```python
from build123d import *
from build123d.topology import SkipClean

# Parameters (mm, degrees)
SKETCH_1_R           = 7.5
SKETCH_1_R_2         = 4.5
EXTRUDE_1_DEPTH      = 125
EXTRUDE_2_REACH      = 151.958
EXTRUDE_2_END_RADIUS = 7.5
SKETCH_2_R           = 7.5
SKETCH_2_R_2         = 4.5
EXTRUDE_3_REACH      = 169.5
EXTRUDE_3_END_RADIUS = 7.5
SKETCH_3_R           = 7.5
SKETCH_3_R_2         = 4.5
SKETCH_4_R           = 7.5
EXTRUDE_4_DEPTH      = 5
EXTRUDE_START        = 5
SKETCH_5_R           = 7.5
EXTRUDE_5_DEPTH      = 5


with BuildPart() as part:
    # 草图1 → 凸台-拉伸1 (new, symmetric)
    with BuildSketch(Plane.XY):
        Circle(SKETCH_1_R)
        Circle(SKETCH_1_R_2, mode=Mode.SUBTRACT)
    extrude(amount=EXTRUDE_1_DEPTH, both=True)

    # 凸台-拉伸2: up to this cylinder (the profile starts outside it)
    extrude_2_end = Plane(origin=(0, 0, -7.287868), z_dir=(0, 0, -1)) * Cylinder(EXTRUDE_2_END_RADIUS, 319.916, mode=Mode.PRIVATE)
    # 草图2 → 凸台-拉伸2 (add, up to the surface)
    with BuildSketch(Plane(origin=(0, 75, 0), x_dir=(1, 0, 0), z_dir=(0, 1, 0)), mode=Mode.PRIVATE) as extrude_2_sk1:
        with Locations(Location((0, 0, 0), (0, 0, 270))):
            Circle(SKETCH_2_R)
        with Locations(Location((0, 0, 0), (0, 0, 270))):
            Circle(SKETCH_2_R_2, mode=Mode.SUBTRACT)
    extrude_2_tool1 = extrude(extrude_2_sk1.sketch, amount=-EXTRUDE_2_REACH, mode=Mode.PRIVATE) - extrude_2_end
    add(extrude_2_tool1.solids().sort_by_distance((0, 75, -7.287868))[0])

    # 凸台-拉伸3: up to this cylinder (the profile starts outside it)
    extrude_3_end = Plane(origin=(0, 0, 0), z_dir=(0, 0, -1)) * Cylinder(EXTRUDE_3_END_RADIUS, 549.575736, mode=Mode.PRIVATE)
    # 草图3 → 凸台-拉伸3 (add, up to the surface)
    with BuildSketch(Plane(origin=(75, 0, 0), x_dir=(0, 0, -1), z_dir=(1, 0, 0)), mode=Mode.PRIVATE) as extrude_3_sk1:
        with Locations((-45, 0)):
            Circle(SKETCH_3_R)
        with Locations((-45, 0)):
            Circle(SKETCH_3_R_2, mode=Mode.SUBTRACT)
    extrude_3_tool1 = extrude(extrude_3_sk1.sketch, amount=-EXTRUDE_3_REACH, mode=Mode.PRIVATE) - extrude_3_end
    add(extrude_3_tool1.solids().sort_by_distance((75, 0, 52.287868))[0])
    # 草图3 → 凸台-拉伸3 (add, up to the surface)
    with BuildSketch(Plane(origin=(75, 0, 0), x_dir=(0, 0, -1), z_dir=(1, 0, 0)), mode=Mode.PRIVATE) as extrude_3_sk2:
        with Locations((-90, 0)):
            Circle(SKETCH_3_R)
        with Locations((-90, 0)):
            Circle(SKETCH_3_R_2, mode=Mode.SUBTRACT)
    extrude_3_tool2 = extrude(extrude_3_sk2.sketch, amount=-EXTRUDE_3_REACH, mode=Mode.PRIVATE) - extrude_3_end
    add(extrude_3_tool2.solids().sort_by_distance((75, 0, 97.287868))[0])
    # 草图3 → 凸台-拉伸3 (add, up to the surface)
    with BuildSketch(Plane(origin=(75, 0, 0), x_dir=(0, 0, -1), z_dir=(1, 0, 0)), mode=Mode.PRIVATE) as extrude_3_sk3:
        with Locations(Location((90, 0, 0), (0, 0, 180))):
            Circle(SKETCH_3_R)
        with Locations((90, 0)):
            Circle(SKETCH_3_R_2, mode=Mode.SUBTRACT)
    extrude_3_tool3 = extrude(extrude_3_sk3.sketch, amount=-EXTRUDE_3_REACH, mode=Mode.PRIVATE) - extrude_3_end
    add(extrude_3_tool3.solids().sort_by_distance((75, 0, -97.287868))[0])
    # 草图3 → 凸台-拉伸3 (add, up to the surface)
    with BuildSketch(Plane(origin=(75, 0, 0), x_dir=(0, 0, -1), z_dir=(1, 0, 0)), mode=Mode.PRIVATE) as extrude_3_sk4:
        with Locations(Location((45, 0, 0), (0, 0, 180))):
            Circle(SKETCH_3_R)
        with Locations((45, 0)):
            Circle(SKETCH_3_R_2, mode=Mode.SUBTRACT)
    extrude_3_tool4 = extrude(extrude_3_sk4.sketch, amount=-EXTRUDE_3_REACH, mode=Mode.PRIVATE) - extrude_3_end
    add(extrude_3_tool4.solids().sort_by_distance((75, 0, -52.287868))[0])

    # 草图4 → 凸台-拉伸4 (add)
    with SkipClean():  # the faces are left unmerged after this step: merging them gives an invalid solid
        with BuildSketch(Plane(origin=(0, 0, -125), x_dir=(-1, 0, 0), z_dir=(0, 0, -1))):
            Circle(SKETCH_4_R)
        extrude(amount=EXTRUDE_4_DEPTH)

    # 草图5 → 凸台-拉伸5 (add)
    with SkipClean():  # the faces are left unmerged after this step: merging them gives an invalid solid
        with BuildSketch(Plane.XY.offset(125).offset(EXTRUDE_START)):
            with Locations(Location((0, 0, 0), (0, 0, 180))):
                Circle(SKETCH_5_R)
        extrude(amount=-EXTRUDE_5_DEPTH)


solid = part.part
```
Geometry check sheet. Reference: the model listing, model coordinates, mm. A direction names the side the tool comes from. Give positions to 0.01 mm unless a question says otherwise; leave off trailing zeros. Write each loop counter-clockwise with the first axis right and the second up, starting at its lowest first coordinate (ties: lowest second). Pieces come first, ordered by that corner, then holes. Notation, with made-up numbers: (42, 17) - (47, 17) arc R17 cw to (47, 36) - close; hole circle Ø4 at (84.5, 3.5). An arc over 180 degrees is marked (long way). Use a Markdown table: item, result.
Q1. Section check A-A, the plane x = 34.5. Enter the section's corners in (y, z), then the cut area to 3 significant figures.
Computed:
| item | result |
|---|---|
| outline | circle Ø15 at (0, -90); circle Ø15 at (0, -45); circle Ø15 at (0, 45); circle Ø15 at (0, 90); hole circle Ø9 at (0, -90); hole circle Ø9 at (0, -45); hole circle Ø9 at (0, 45); hole circle Ø9 at (0, 90) |
| area | 452 mm² |
Q2. Go/stop test with flat-tipped pins: P1, Ø11.5, axis at y = 0, z = 90, coming from the +X side; P2, Ø6, axis at x = 11, z = -53, coming from the +Y side; P3, Ø2, axis at x = 46, z = 89.5, coming from the +Y side; P4, Ø6, axis at x = 5.5, y = 14, coming from the -Z side. Record where each tip stops, or that it passes through.
Computed:
| item | result |
|---|---|
| P1 | stops at x = 75 |
| P2 | stops at y = 5.59 |
| P3 | stops at y = 7.5 |
| P4 | stops at z = -7.07 |
Q3. Thickness scan on L1, parallel to Y at x = 0, z = 37; L2, parallel to Z at x = 26.5, y = 5.5; L3, parallel to X at y = 26, z = -0.5. Record the ranges inside material, lowest first. Write a range as [from, to].
Computed:
| item | result |
|---|---|
| L1 | y = [-7.5, -4.5], [4.5, 7.5] |
| L2 | z = [-95.1, -84.9], [-50.1, -39.9], [39.9, 50.1], [84.9, 95.1] |
| L3 | x = [-7.48, -4.47], [4.47, 7.48] |
Q4. Section check C-C, the plane y = 48.5. Enter the section's corners in (x, z), then the cut area to 3 significant figures.
Computed:
| item | result |
|---|---|
| outline | circle Ø15 at (0, 0); hole circle Ø9 at (0, 0) |
| area | 113 mm² |
Q5. Section check B-B, the plane z = 45. Enter the section's corners in (x, y).
Computed:
| item | result |
|---|---|
| outline | (0, -7.5) - (75, -7.5) - (75, -4.5) - (6, -4.5) arc R7.5 ccw to (6, 4.5) - (75, 4.5) - (75, 7.5) - (0, 7.5) arc R7.5 ccw to start; hole circle Ø9 at (0, 0) |
Q6. Draft check along Y on faces 6 (the face through (40.983, 1.352, -49.292)), 7 (the face through (-5, 75, 0)), 8 (the face through (75, -5, 45)), 9 (the face through (38.025, 2.253, 82.846)). Enter one of: pulls with the +Y half, pulls with the -Y half, needs draft (parallel to the pull), parting line crosses it, or undercut.
Computed:
| item | result |
|---|---|
| face 6 | undercut |
| face 7 | pulls with the +Y half |
| face 8 | needs draft |
| face 9 | parting line crosses it |
Q7. Set-up check for faces 1 (the face through (1.352, 40.983, 4.292)), 2 (the face through (75, -5, 90)), 3 (the face through (0, 0, -125)), 4 (the face through (0, 0, 130)), 5 (the face through (40.983, 1.352, 40.708)): record each of +Z, -Z, +X, -X, +Y, -Y from which the full face is reachable in a straight line by a thin tool's end or side.
Computed:
| item | result |
|---|---|
| face 1 | +Y |
| face 2 | +Z, -Z, +X, +Y, -Y |
| face 3 | none |
| face 4 | +Z, +X, -X, +Y, -Y |
| face 5 | +X |
